Input: part model. Units: mm. Frame: model coordinates. Coordinates: 2 decimals unless noted, no trailing zeros. Order: outer loops, then holes, each group sorted by start corner. A loop starts at its lowest first (then second) coordinate and runs counter-clockwise, first axis right, second up. Notation, with made-up numbers: (75.5, 61.25) -> (108.5, 61.25) arc R28 ccw to (108.5, 80.25) -> close; hole circle Ø10 at (-4, -1.5). An arc over 180 degrees is marked (long way). Use one line per item in the form item = value. Start each with the question number.
1) Draft query along X for faces 1 (the flat face through (-5.76, 1.01, 58.02)), 2 (the flat face through (11.824, 0.986, 113.374)), 3 (the cylindrical face through (21.26, 0.99, -20.14)). Return one class per face: pulls with the +X half, pulls with the -X half, needs draft (parallel to the pull), parting line crosses it, or undercut.
2) Pin query (flat end, axial travel): pin 1 (1 mm diameter, centred on x = -47.5, y = 1, fed in from +Z); pin 2 (1 mm diameter, centred on x = 10, y = 1.5, fed in from +Z). Return the tip coordinate at first contact, or that it passes through.
3) Section query B-B on x = -24. Output: boundary loops of the cut face in (y, z), then the cut area to 3 significant figures.
4) Section query A-A on y = 0.6. Count the separate pieces of the cut face and the enclosed holes in it, then the cut area to 3 significant figures.
5) Section query C-C on z = 20. Output: boundary loops of the cut face in (x, y), then the cut area to 3 significant figures.
6) Ray query, line 1 along X through (y, z) = (0.65, 77.5); line 2 along Z through (x, y) = (-36, 1.05); line 3 along Z through (x, y) = (-13.5, 1.35). Return the intervals inside material, ascending.
from build123d import *

# Parameters (mm, degrees)
SKETCH_1_R               = 1.75
EXTRUDE_1_DEPTH          = 2
SKETCH_4_W               = 29
SKETCH_4_H               = 65
SKETCH_4_R               = 3.5
EXTRUDE_2_DEPTH          = 2
SKETCH_5_R               = 19.2
CUT_EXTRUDE_1_DEPTH      = 1
CUT_EXTRUDE_1_DEPTH_BACK = 3
CUT_EXTRUDE_2_DEPTH      = 1
CUT_EXTRUDE_2_DEPTH_BACK = 3
FILLET_1_R               = 3
SKETCH_9_R               = 1.5
CUT_EXTRUDE_4_DEPTH      = 1
CUT_EXTRUDE_4_DEPTH_BACK = 3
FILLET_2_R               = 1
SKETCH_13_R              = 1.25
CUT_EXTRUDE_6_DEPTH      = 1
CUT_EXTRUDE_6_DEPTH_BACK = 3
SKETCH_15_R              = 1.25
CUT_EXTRUDE_7_DEPTH      = 1
CUT_EXTRUDE_7_DEPTH_BACK = 3


with BuildPart() as part:
    # Эскиз1 → Бобышка-Вытянуть1 (new body)
    with BuildSketch(Plane(origin=(0, 0, 0), x_dir=(1, 0, 0), z_dir=(0, 1, 0))):
        Polygon((-57.045428332, 34.194915254), (32.954571668, 34.194915254), (32.954571668, -95.805084746), (-11.545428332, -132.805084746), (-11.545428332, -55.805084746), (17.454571668, -55.805084746), (17.454571668, 9.194915254), (-57.045428332, 9.194915254), align=None)
        with Locations((-44.545428332, 21.694915254)):
            Circle(SKETCH_1_R, mode=Mode.SUBTRACT)
        with Locations((-12.045428332, 21.694915254)):
            Circle(SKETCH_1_R, mode=Mode.SUBTRACT)
        with Locations((20.454571668, 21.694915254)):
            Circle(SKETCH_1_R, mode=Mode.SUBTRACT)
        with Locations((20.454571668, -10.805084746)):
            Circle(SKETCH_1_R, mode=Mode.SUBTRACT)
        with Locations((20.454571668, -43.305084746)):
            Circle(SKETCH_1_R, mode=Mode.SUBTRACT)
    extrude(amount=EXTRUDE_1_DEPTH)

    # Эскиз4 → Бобышка-Вытянуть2 (add)
    with BuildSketch(Plane(origin=(0, 2, 0), x_dir=(1, 0, 0), z_dir=(0, 1, 0))):
        with Locations((2.954571668, -23.305084746)):
            Rectangle(SKETCH_4_W, SKETCH_4_H)
        with Locations((12.027100485, -48.375084746)):
            Circle(SKETCH_4_R, mode=Mode.SUBTRACT)
        with Locations((11.493153901, -1.266502513)):
            Circle(SKETCH_4_R, mode=Mode.SUBTRACT)
    extrude(amount=-EXTRUDE_2_DEPTH)

    # Эскиз5 → Вырез-Вытянуть1 (cut, two sides)
    with BuildSketch(Plane(origin=(0, 2, 0), x_dir=(1, 0, 0), z_dir=(0, 1, 0))) as cut_extrude_1_sk:
        with Locations((-12.045428332, -24.805084746)):
            Circle(SKETCH_5_R)
    extrude(amount=CUT_EXTRUDE_1_DEPTH, mode=Mode.SUBTRACT)
    extrude(cut_extrude_1_sk.sketch, amount=-CUT_EXTRUDE_1_DEPTH_BACK, mode=Mode.SUBTRACT)

    # Эскиз7 → Вырез-Вытянуть2 (cut, two sides)
    with BuildSketch(Plane(origin=(0, 2, 0), x_dir=(1, 0, 0), z_dir=(0, 1, 0))) as cut_extrude_2_sk:
        with BuildLine():
            Line((-0.545428332, -40.180064421), (-11.545428332, -77.80926144))
            Line((-11.545428332, -77.80926144), (-11.545428332, -43.998573225))
            ThreePointArc((-11.545428332, -43.998573225), (-5.751853603, -42.935021213), (-0.545428332, -40.180064421))
        make_face()
    extrude(amount=CUT_EXTRUDE_2_DEPTH, mode=Mode.SUBTRACT)
    extrude(cut_extrude_2_sk.sketch, amount=-CUT_EXTRUDE_2_DEPTH_BACK, mode=Mode.SUBTRACT)

    # Скругление1
    fillet_1_edges = [part.edges().sort_by_distance(p)[0] for p in [
        (-57.045428332, 1, -34.194915254),
        (32.954571668, 1, -34.194915254),
    ]]
    fillet(fillet_1_edges, radius=FILLET_1_R)

    # Эскиз9 → Вырез-Вытянуть4 (cut, two sides)
    with BuildSketch(Plane(origin=(0, 2, 0), x_dir=(1, 0, 0), z_dir=(0, 1, 0))) as cut_extrude_4_sk:
        with Locations((-11.545428332, -77.80926144)):
            Circle(SKETCH_9_R)
    extrude(amount=CUT_EXTRUDE_4_DEPTH, mode=Mode.SUBTRACT)
    extrude(cut_extrude_4_sk.sketch, amount=-CUT_EXTRUDE_4_DEPTH_BACK, mode=Mode.SUBTRACT)

    # Скругление2
    fillet_2_edges = [part.edges().sort_by_distance(p)[0] for p in [
        (-11.545428332, 1, 132.805084746),
    ]]
    fillet(fillet_2_edges, radius=FILLET_2_R)

    # Эскиз13 → Вырез-Вытянуть6 (cut, two sides)
    with BuildSketch(Plane(origin=(0, 2, 0), x_dir=(1, 0, 0), z_dir=(0, 1, 0))) as cut_extrude_6_sk:
        with Locations((-9.54492596, -95.551225642)):
            Circle(SKETCH_13_R)
        with Locations((-9.54492596, -117.508337259)):
            Circle(SKETCH_13_R)
    extrude(amount=CUT_EXTRUDE_6_DEPTH, mode=Mode.SUBTRACT)
    extrude(cut_extrude_6_sk.sketch, amount=-CUT_EXTRUDE_6_DEPTH_BACK, mode=Mode.SUBTRACT)

    # Эскиз15 → Вырез-Вытянуть7 (cut, two sides)
    with BuildSketch(Plane(origin=(0, 2, 0), x_dir=(1, 0, 0), z_dir=(0, 1, 0))) as cut_extrude_7_sk:
        with Locations((-1.545428332, -117.398618322)):
            Circle(SKETCH_15_R)
        with Locations((-1.545428332, -97.398618322)):
            Circle(SKETCH_15_R)
        with Locations((-1.545428332, -77.398618322)):
            Circle(SKETCH_15_R)
    extrude(amount=CUT_EXTRUDE_7_DEPTH, mode=Mode.SUBTRACT)
    extrude(cut_extrude_7_sk.sketch, amount=-CUT_EXTRUDE_7_DEPTH_BACK, mode=Mode.SUBTRACT)


solid = part.part
Answers below:
q1.face_1 = pulls with the -X half
q1.face_2 = pulls with the +X half
q1.face_3 = undercut
q2.pin_1 = -9.19
q2.pin_2 = 115.31
q3.outline = (0, -34.19) -> (2, -34.19) -> (2, -9.19) -> (0, -9.19) -> close
q3.area = 50.0 mm^2
q4.separate_pieces = 1
q4.enclosed_holes = 12
q4.area = 6,850 mm^2
q5.outline = (6.54, 0) -> (32.95, 0) -> (32.95, 2) -> (6.54, 2) -> close
q5.area = 52.8 mm^2
q6.line_1 = -10.08 to -2.79, -0.3 to 32.95
q6.line_2 = -34.19 to -9.19
q6.line_3 = -34.19 to -22.67, -20.72 to -9.19
